Verification items for the finished model (mm, model axes). Give positions to 0.01 mm unless a question says otherwise; leave off trailing zeros. Order: outer loops, then holes, each group sorted by start corner. A loop starts at its lowest first (then second) coordinate and runs counter-clockwise, first axis right, second up. Notation, with made-up numbers: (48.5, 2.25) -> (83.5, 2.25) arc R32 ccw to (83.5, 41.25) -> close; hole circle Ø8 at (74, -2.75). An arc over 180 degrees is marked (long way). Write each question's results on one line, items separated by ' | '. Start each with the question number.
1. Cross-section at D-D, the plane x = -25.9. Enter the section's corners in (y, z).
2. Mould release check, pull along X, two halves, no side actions. Record for faces 1 (the face through (-26, -15, 2)), 2 (the face through (-53.5, 11.43, 2.46)), 3 (the face through (5, 0, 2)): +X half, -X half, draft (parallel to the pull), parting line (faces both ways), or undercut.
3. Cross-section at A-A, the plane x = 0. Enter the section's corners in (y, z).
4. Cross-section at B-B, the plane z = 2.8. Enter the section's corners in (x, y).
5. Cross-section at C-C, the plane y = 0. Enter the section's corners in (x, z), then the cut area to 4 significant figures.
6. Depth check by flat-ended pin: pin 1 Ø15.5 at (x, y) = (-25.9, 0) entering from -Z. Enter the tip coordinate at first touch or a pass-through.
7. Material ranges on L1, parallel to Y at x = -51.8, z = 3.2; L2, parallel to X at y = -11, z = 1.4; L3, parallel to X at y = 12.5, z = 0.75, recorded low to high. Write a range as from..to.
Autodesk Inventor part; units mm, degrees
ref_plane "YZ Plane" through (0, 0, 0) normal (1, 0, 0) x (0, 1, 0)
ref_plane "XZ Plane" through (0, 0, 0) normal (0, 1, 0) x (-1, 0, 0)
ref_plane "XY Plane" through (0, 0, 0) normal (0, 0, 1) x (1, 0, 0)
sketch "Sketch1" plane through (0, 0, 0) normal (0, 0, 1) x (1, 0, 0)
  circle A0 centre (0, -32.5) radius 1.7
  circle A1 centre (0, 11.5) radius 1.7
  circle A2 centre (0, -11.5) radius 1.7
  line L0 (5, 15) -> (-5, 15)
  line L1 (-5, 15) -> (-5, -15)
  line L2 (-5, -15) -> (5, -15)
  line L3 (5, -15) -> (5, 15)
  circle A3 centre (-51.8, 11.5) radius 1.7
  circle A4 centre (-51.8, -11.5) radius 1.7
  line L4 (-46.8, 15) -> (-56.8, 15)
  line L5 (-56.8, 15) -> (-56.8, -15)
  line L6 (-56.8, -15) -> (-46.8, -15)
  line L7 (-46.8, -15) -> (-46.8, 15)
  line L8 (-56.8, 15) -> (5, 15)
  line L9 (5, 15) -> (5, -15)
  line L10 (5, -15) -> (-56.8, -15)
  line L11 (-56.8, -15) -> (-56.8, 15)
  line L12 (-5, 0) -> (-46.8, 0) construction
  line L13 (-25.9, -15) -> (-25.9, 15) construction
  circle A5 centre (-25.9, 0) radius 8.65
  point P0 (0, 0)
  point P1 (-5, 15)
  point P2 (-46.8, 15)
  point P3 (-46.8, -15)
  point P4 (-5, -15)
  point P5 (-46.8, -15)
  point P6 (-56.8, -15)
  point P7 (-5, 15)
  point P8 (-46.8, 15)
  point P9 (-56.8, -15)
  dimension "d0" = 17.3
extrude "Extrusion1" add sketch "Sketch1" along normal blind 5 contours L3 L2 L1 L0 | L1 L10 L7 L8 | L7 L6 L5 L4
properties part number "CenterPointBracket"
Results below:
1) outline: (-15, 0) -> (-8.65, 0) -> (-8.65, 5) -> (-15, 5) -> close; (8.65, 0) -> (15, 0) -> (15, 5) -> (8.65, 5) -> close
2) face 1: draft | face 2: undercut | face 3: +X half
3) outline: (-15, 0) -> (-13.2, 0) -> (-13.2, 5) -> (-15, 5) -> close; (-9.8, 0) -> (9.8, 0) -> (9.8, 5) -> (-9.8, 5) -> close; (13.2, 0) -> (15, 0) -> (15, 5) -> (13.2, 5) -> close
4) outline: (-56.8, -15) -> (5, -15) -> (5, 15) -> (-56.8, 15) -> close; hole circle Ø3.4 at (-51.8, -11.5); hole circle Ø3.4 at (-51.8, 11.5); hole circle Ø17.3 at (-25.9, 0); hole circle Ø3.4 at (0, -11.5); hole circle Ø3.4 at (0, 11.5)
5) outline: (-56.8, 0) -> (-34.55, 0) -> (-34.55, 5) -> (-56.8, 5) -> close; (-17.25, 0) -> (5, 0) -> (5, 5) -> (-17.25, 5) -> close | area: 222.5 mm²
6) pin 1: passes through
7) L1: y = -15..-13.2, -9.8..9.8, 13.2..15 | L2: x = -56.8..-53.42, -50.18..-1.62, 1.62..5 | L3: x = -56.8..-53.17, -50.43..-1.37, 1.37..5
